from build123d import *

# Parameters (mm, degrees)
EXTRUDE2_DEPTH      = 1.25
SKETCH3_R           = 5
EXTRUDE1_DEPTH      = 0.55566
EXTRUDE1_DRAFT      = -5
SKETCH15_R          = 4.951386049
EXTRUDE3_DEPTH      = 3.14874
EXTRUDE3_TAPER      = 26.698437176
FILLET3_R           = 0.254
SKETCH4_R           = 2.5
CUT_EXTRUDE1_DEPTH  = 16.684929072
SWEEP1_PITCH        = 0.8
SKETCH7_R           = 5
CUT_EXTRUDE2_DEPTH  = 16.684929104
SKETCH8_R           = 4.951386049
CUT_EXTRUDE3_DEPTH  = 14.546328962
SKETCH11_R          = 2.4492
CUT_EXTRUDE5_DEPTH  = 14.546328926
CUT_EXTRUDE5_TAPER  = 45
CHAMFER1_SIZE       = 0.2083725
CHAMFER1_SIZE2      = 0.192340809
FILLET4_R           = 0.416666667
SKETCH18_R          = 3.211270087
BOSS_EXTRUDE3_DEPTH = 3.7044
SKETCH19_R          = 2.5
CUT_EXTRUDE6_DEPTH  = 3.7044
CHAMFER2_SIZE       = 0.2


with BuildPart() as part:
    # Sketch13 → Extrude2 (new, symmetric)
    with BuildSketch(Plane(origin=(0, 0, 0), x_dir=(1, 0, 0), z_dir=(0, 1, 0))):
        with BuildLine():
            Line((3.074810737, 0.27783), (5, 0.27783))
            ThreePointArc((5, 0.27783), (7.099129938, 0.776746992), (8.749295866, 2.166789103))
            ThreePointArc((8.749295866, 2.166789103), (10.222034162, 5.009156698), (10.73, 8.169850029))
            ThreePointArc((10.73, 8.169850029), (10.648713606, 8.495871948), (10.423883961, 8.745570566))
            ThreePointArc((10.423883961, 8.745570566), (8.013491694, 9.895268701), (5.372282902, 10.29))
            ThreePointArc((5.372282902, 10.29), (4.94953191, 10.146495375), (4.701501078, 9.775291004))
            Line((4.701501078, 9.775291004), (3.074810737, 3.7044))
            Line((3.074810737, 3.7044), (3.074810737, 0.27783))
        make_face()
    extrude(amount=EXTRUDE2_DEPTH, both=True)

    # Fillet4
    fillet4_edges = [part.edges().sort_by_distance(p)[0] for p in [
        (7.099129938, 1.25, -0.776746992),
        (10.222034162, 1.25, -5.009156698),
        (10.648713606, 1.25, -8.495871948),
        (8.013491694, 1.25, -9.895268701),
        (4.94953191, 1.25, -10.146495375),
        (3.888155907, 1.25, -6.739845502),
        (3.888155907, -1.25, -6.739845502),
        (4.037405368, 1.25, -0.27783),
        (4.94953191, -1.25, -10.146495375),
        (8.013491694, -1.25, -9.895268701),
        (10.648713606, -1.25, -8.495871948),
        (10.222034162, -1.25, -5.009156698),
        (7.099129938, -1.25, -0.776746992),
        (4.037405368, -1.25, -0.27783),
    ]]
    fillet(fillet4_edges, radius=FILLET4_R)


with BuildPart() as body_2:
    # Sketch3 → Extrude1 (with draft: the straight prism first)
    with BuildSketch(Plane.XY):
        Circle(SKETCH3_R)
    extrude(amount=-EXTRUDE1_DEPTH)
    # Extrude1: the draft: its side faces are tilted about the plane it starts from
    extrude1_sides = [body_2.faces().sort_by_distance(p)[0] for p in [
        (-5, 0, -0.27783),
    ]]
    draft(extrude1_sides, Plane.XY, EXTRUDE1_DRAFT)

    # Sketch15 → Extrude3 (add)
    with BuildSketch(Plane(origin=(0, 0, -0.55566), x_dir=(-1, 0, 0), z_dir=(0, 0, -1))):
        Circle(SKETCH15_R)
    extrude(amount=EXTRUDE3_DEPTH, taper=EXTRUDE3_TAPER)

    # Fillet3
    fillet3_edges = [body_2.edges().sort_by_distance(p)[0] for p in [
        (3.367842423, 0, -3.7044),
    ]]
    fillet(fillet3_edges, radius=FILLET3_R)

    # Sketch4 → Cut-Extrude1 (cut, through all)
    with BuildSketch(Plane.XY):
        Circle(SKETCH4_R)
    extrude(amount=-CUT_EXTRUDE1_DEPTH, mode=Mode.SUBTRACT)

    # Sweep1: the profile of Sketch6 profile screwed along a right-hand helix of 7.1305 turns, 6 arcs to a turn; built about Z, then put on its axis
    sweep1_z = Axis((0, 0, 0), (0, 0, 1))
    sweep1_corners = [(2.5003, 0, -0.700173205), (1.980384758, 0, -0.4), (1.980384758, 0, -0.3), (2.5003, 0, 0.000173205)]
    with BuildLine(mode=Mode.PRIVATE) as sweep1_profile:
        Line(sweep1_corners[0], sweep1_corners[1])
        Line(sweep1_corners[1], sweep1_corners[2])
        Line(sweep1_corners[2], sweep1_corners[3])
        Line(sweep1_corners[3], sweep1_corners[0])
    sweep1_cap = Face(sweep1_profile.wire())
    sweep1_turn_angles = [0, 30, 60, 90, 120, 150, 180, 210, 240, 270, 300, 330, 360]
    sweep1_turn_weights = [1, 0.8660254037844387, 1, 0.8660254037844387, 1, 0.8660254037844387, 1, 0.8660254037844387, 1, 0.8660254037844387, 1, 0.8660254037844387, 1]
    sweep1_turn_rails = [Edge.make_bspline([Vector(p[0], p[1], 0).rotate(sweep1_z, sweep1_turn_angles[k]) / sweep1_turn_weights[k] + Vector(0, 0, p[2] + SWEEP1_PITCH * sweep1_turn_angles[k] / 360) for k in range(13)], [0, 0, 0, 1, 1, 2, 2, 3, 3, 4, 4, 5, 5, 6, 6, 6], 2, sweep1_turn_weights) for p in sweep1_corners]
    sweep1_turn_sides = [Face.make_surface_from_curves(sweep1_turn_rails[p[0]], sweep1_turn_rails[p[1]]) for p in [(0, 1), (1, 2), (2, 3), (3, 0)]]
    sweep1_last_angles = [2520, 2543.49, 2566.98]
    sweep1_last_weights = [1, 0.9171296552585544, 1]
    sweep1_last_rails = [Edge.make_bspline([Vector(p[0], p[1], 0).rotate(sweep1_z, sweep1_last_angles[k]) / sweep1_last_weights[k] + Vector(0, 0, p[2] + SWEEP1_PITCH * sweep1_last_angles[k] / 360) for k in range(3)], [0, 0, 0, 1, 1, 1], 2, sweep1_last_weights) for p in sweep1_corners]
    sweep1_last_sides = [Face.make_surface_from_curves(sweep1_last_rails[p[0]], sweep1_last_rails[p[1]]) for p in [(0, 1), (1, 2), (2, 3), (3, 0)]]
    sweep1 = Plane(origin=(0, 0, 0), x_dir=(-1, 0, 0), z_dir=(0, 0, -1)) * Solid(Shell([*[p.moved(Location((0, 0, SWEEP1_PITCH * i))) for i in range(7) for p in sweep1_turn_sides], *sweep1_last_sides, sweep1_cap, sweep1_cap.rotate(sweep1_z, 2566.98).moved(Location((0, 0, SWEEP1_PITCH * 2566.98 / 360)))]))
    add(sweep1)

    # Sketch7 → Cut-Extrude2 (cut, through all)
    with BuildSketch(Plane.XY):
        Circle(SKETCH7_R)
    extrude(amount=CUT_EXTRUDE2_DEPTH, mode=Mode.SUBTRACT)

    # Sketch8 → Cut-Extrude3 (cut, through all)
    with BuildSketch(Plane.XY.offset(-3.7044)):
        Circle(SKETCH8_R)
    extrude(amount=-CUT_EXTRUDE3_DEPTH, mode=Mode.SUBTRACT)

    # Cut-Extrude4 cone 1 section (through the dimple's axis) → Cut-Extrude4 (revolve, cut)
    with BuildSketch(Plane(origin=(0, 0, 0), x_dir=(0, -1, 0), z_dir=(1, 0, 0))):
        Polygon((0, 0), (2.5, 0), (0, 2.5), align=None)
    revolve(axis=Axis((0, 0, 0), (0, 0, -1)), mode=Mode.SUBTRACT)

    # Sketch11 → Cut-Extrude5 (cut, through all)
    with BuildSketch(Plane.XY.offset(-3.7044)):
        Circle(SKETCH11_R)
    extrude(amount=CUT_EXTRUDE5_DEPTH, taper=CUT_EXTRUDE5_TAPER, mode=Mode.SUBTRACT)

    # Chamfer1
    chamfer1_edges = [body_2.edges().sort_by_distance(p)[0] for p in [
        (-5, 0, 0),
    ]]
    chamfer1_side = [body_2.faces().sort_by_distance(p)[0] for p in [
        (-4.975693025, 0, -0.27783),
    ]]
    chamfer(chamfer1_edges, length=CHAMFER1_SIZE, length2=CHAMFER1_SIZE2, reference=chamfer1_side[0])


with BuildPart() as body_3:
    # Mirror6: mirrored copy
    add(part.part.mirror(Plane(origin=(0, 0, 0), x_dir=(0, 0, 1), z_dir=(1, 0, 0))))

    # Combine2: union part, body 2
    add(part.part)
    add(body_2.part)

    # Sketch18 → Boss-Extrude3 (add)
    with BuildSketch(Plane(origin=(0, 0, -3.7044), x_dir=(-1, 0, 0), z_dir=(0, 0, -1))):
        Circle(SKETCH18_R)
    extrude(amount=-BOSS_EXTRUDE3_DEPTH)

    # Sketch19 → Cut-Extrude6 (cut)
    with BuildSketch(Plane(origin=(0, 0, -3.7044), x_dir=(-1, 0, 0), z_dir=(0, 0, -1))):
        Circle(SKETCH19_R)
    extrude(amount=-CUT_EXTRUDE6_DEPTH, mode=Mode.SUBTRACT)

    # Chamfer2
    chamfer2_edges = [body_3.edges().sort_by_distance(p)[0] for p in [
        (2.5, 0, -3.7044),
        (2.5, 0, 0),
    ]]
    chamfer(chamfer2_edges, length=CHAMFER2_SIZE)


solid = body_3.part
Read the model definition and answer for the solid it produces. Units are mm, in the model's axes. A direction names the side the tool comes from. Round coordinates to 2 decimals unless told otherwise and drop trailing zeros. Write each loop counter-clockwise with the first axis right and the second up, starting at its lowest first coordinate (ties: lowest second). Pieces come first, ordered by that corner, then holes.
Q1. Find section A-A on x = 0. Determine the outline of the cut face in (y, z).
Values:
outline: (-4.98, -0.21) - (-4.95, -0.56) - (-3.44, -3.56) arc R0.25 ccw to (-3.21, -3.7) - (-2.7, -3.7) - (-2.5, -3.5) - (-2.5, -0.2) - (-2.7, 0) - (-4.81, 0) - close; (2.5, -3.5) - (2.7, -3.7) - (3.21, -3.7) arc R0.25 ccw to (3.44, -3.56) - (4.95, -0.56) - (4.98, -0.21) - (4.81, 0) - (2.7, 0) - (2.5, -0.2) - close
Q2. The mould has two halves that part along X. Classify faces 1 (the face through (3.949, 1.131, -6.481)), 2 (the face through (-8, 0, -9.9)), 3 (the face through (7, 1.25, -5)): released by +X, released by -X, zero draft, split by the parting line, or undercut.
Values:
face 1: undercut
face 2: released by -X
face 3: zero draft
Q3. Flat-ended cylindrical pins translate along their axes: P1, Ø1, axis at y = 1, z = -4, coming from the -X side; P2, Ø1.5, axis at x = -6, z = -6.5, coming from the -Y side; P3, Ø1, axis at x = -5, y = 2, coming from the +Z side. Find the tip coordinate at first contact, or state that the pin passes through.
Values:
P1: stops at x = -10.03
P2: stops at y = -1.25
P3: stops at z = -0.09
Q4. Straight lines are drawn through the part: line 1 (Y direction, x = 0, z = -2.25); line 2 (Y direction, x = 0, z = -0.9); line 3 (X direction, y = 1, z = -3.25). For each, find the intervals that lie inside material, in ascending order.
Values:
line 1: y = -4.1 to -2.5, 2.5 to 4.1
line 2: y = -4.78 to -2.5, 2.5 to 4.78
line 3: x = -9.41 to -2.29, 2.29 to 9.41
Q5. A tool of negligible diameter and unlimited length cuts with its end or side. For faces 4 (the face through (7, -1.25, -5)), 5 (the face through (3.942, -1.125, -6.483)), 6 (the face through (-7, -1.25, -5)), from which of +Z, -Z, +X, -X, +Y, -Y can it reach the whole face along a straight path? Write none if from no direction.
Values:
face 4: -Z, +X, -Y
face 5: -Z, -Y
face 6: -Z, -X, -Y
